from build123d import *

# Parameters (mm, degrees)
F1_DEPTH = 7.5
F2_R     = 4.99999


# Not quite as in the source:
# - a fillet or chamfer is up to 0.001 mm smaller than in the source, because OpenCascade refuses the exact size


with BuildPart() as f1:
    # F0 (on Top) → F1 (new body, symmetric)
    with BuildSketch(Plane.XY):
        with BuildLine():
            ThreePointArc((-68.4076752503, 15.1665699541), (-64.0142769681, 4.5599682363), (-53.4076752503, 0.1665699541))
            Line((-53.4076752503, 0.1665699541), (36.5923247497, 0.1665699541))
            ThreePointArc((36.5923247497, 0.1665699541), (47.1989264675, 4.5599682363), (51.5923247497, 15.1665699541))
            Line((51.5923247497, 15.1665699541), (51.5923247497, 40.1665699541))
            Line((51.5923247497, 40.1665699541), (41.5923247497, 40.1665699541))
            Line((41.5923247497, 40.1665699541), (41.5923247497, 25.1665699541))
            ThreePointArc((41.5923247497, 25.1665699541), (38.6633925615, 18.0955021423), (31.5923247497, 15.1665699541))
            Line((31.5923247497, 15.1665699541), (-48.4076752503, 15.1665699541))
            ThreePointArc((-48.4076752503, 15.1665699541), (-55.4787430622, 18.0955021423), (-58.4076752503, 25.1665699541))
            Line((-58.4076752503, 25.1665699541), (-58.4076752503, 40.1665699541))
            Line((-58.4076752503, 40.1665699541), (-68.4076752503, 40.1665699541))
            Line((-68.4076752503, 40.1665699541), (-68.4076752503, 15.1665699541))
        make_face()
    extrude(amount=F1_DEPTH, both=True)

    # F2 (radius 5 in the source; OpenCascade refuses exactly that, so slightly less here)
    f2_edges = [f1.edges().sort_by_distance(p)[0] for p in [
        (-8.407675, 15.16657, 7.5),
        (-8.407675, 0.16657, 7.5),
        (-8.407675, 0.16657, -7.5),
        (-8.407675, 15.16657, -7.5),
    ]]
    fillet(f2_edges, radius=F2_R)


solid = f1.part
For this review, take the finished solid that the model builds, in its own axes (mm). A direction names the side the tool comes from. Give positions to 0.01 mm unless a question says otherwise; leave off trailing zeros. Loops run counter-clockwise (first coordinate to the right, second up) from the corner with the lowest first, then second, coordinate; pieces in that order, holes last.
Item 1: Take a section at C-C, the plane z = -6. State the section outline as (x, y) points, and give its area (3 significant figures).
Item 2: Take a section at D-D, the plane z = 4.5. State the section outline as (x, y) points.
Item 3: Tool access review of faces 5 (the cylindrical face through (-64.13, 4.677, 0.035)), 6 (the cylindrical face through (-8.97, 13.74, -6)), 7 (the cylindrical face through (43.02, 32.56, 6)), 8 (the flat face through (-9, 8, -7.5)), 9 (the flat face through (-8, 15.167, 0)): name each direction out of +Z, -Z, +X, -X, +Y, -Y from which nothing blocks a thin tool from reaching the whole face with its end or side.
Item 4: Take a section at B-B, the plane x = 27. State the section outline as (y, z) points.
Item 5: For line 1 along X through (y, z) = (37, 2); line 2 along X through (y, z) = (23, 6.25); line 3 along Z through (x, y) = (46.5, 29), list the stretches that pass through material, from the lowest coordinate up.
Item 6: Insertion check: pin 1 (5 mm diameter, centred on x = 29, z = -5.5, fed in from +Y); pin 2 (6 mm diameter, centred on x = 37.5, z = 3.5, fed in from +Y); pin 3 (1.5 mm diameter, centred on x = -24.5, z = -4.5, fed in from -Y). Each pin has a flat end and moves straight along its axis. Give the tip position at first contact, or say it passes through.
Item 7: Draft analysis for pull direction X (two halves, no side actions). For faces 1 (the flat face through (-68.408, 28, 0)), 2 (the cylindrical face through (-8.97, 13.74, 6)), 3 (the flat face through (47, 40.167, 0)), 4 (the cylindrical face through (-59.833, 32.772, 5.996)), state which applies: +X half, -X half, draft (parallel to the pull), parting line (faces both ways), or undercut.
Calculated:
1. outline: (-66.98, 15.17) arc R13.57 ccw to (-53.41, 1.6) - (36.59, 1.6) arc R13.57 ccw to (50.16, 15.17) - (50.16, 40.17) - (43.02, 40.17) - (43.02, 25.17) arc R11.43 cw to (31.59, 13.74) - (-48.41, 13.74) arc R11.43 cw to (-59.84, 25.17) - (-59.84, 40.17) - (-66.98, 40.17) - close
1. area: 1,780 mm2
2. outline: (-67.99, 15.17) arc R14.58 ccw to (-53.41, 0.58) - (36.59, 0.58) arc R14.58 ccw to (51.17, 15.17) - (51.17, 40.17) - (42.01, 40.17) - (42.01, 25.17) arc R10.42 cw to (31.59, 14.75) - (-48.41, 14.75) arc R10.42 cw to (-58.83, 25.17) - (-58.83, 40.17) - (-67.99, 40.17) - close
3. face 5: +Z, -Z, -X, -Y
3. face 6: -Z, +Y
3. face 7: +Z, +Y
3. face 8: -Z, +X, -X, +Y, -Y
3. face 9: +Z, -Z, +Y
4. outline: (0.17, -2.5) arc R5 ccw to (5.17, -7.5) - (10.17, -7.5) arc R5 ccw to (15.17, -2.5) - (15.17, 2.5) arc R5 ccw to (10.17, 7.5) - (5.17, 7.5) arc R5 ccw to (0.17, 2.5) - close
5. line 1: x = -68.41 to -58.41, 41.59 to 51.59
5. line 2: x = -66.71 to -59.9, 43.08 to 49.9
5. line 3: z = -7.5 to 7.5
6. pin 1: stops at y = 15.14
6. pin 2: stops at y = 20.49
6. pin 3: stops at y = 0.33
7. face 1: -X half
7. face 2: undercut
7. face 3: draft
7. face 4: undercut
